The listing builds one solid part. Answer for the finished solid, in the listing's coordinates (mm). Face numbers are marked on the shaded views. A direction names the side the tool comes from. Give positions to 0.01 mm unless a question says otherwise; leave off trailing zeros. Loops run counter-clockwise (first coordinate to the right, second up) from the corner with the lowest first, then second, coordinate; pieces in that order, holes last. Notation, with made-up numbers: (42.25, -18) - (73.25, -18) arc R15 cw to (73.25, 11) - close; hole circle Ø8 at (85, 51). An arc over 180 degrees is marked (long way). Answer in a Markdown table with one row per item. Add a question column.
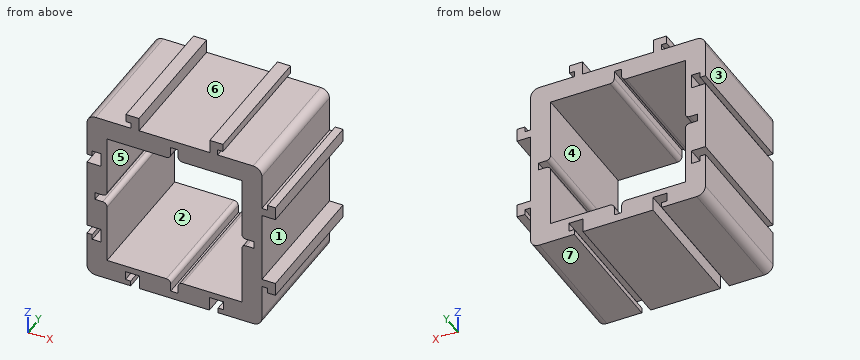
```python
from build123d import *

# Parameters (mm, degrees)
SKETCH1_W           = 50.8
SKETCH1_H           = 50.8
BOSS_EXTRUDE1_DEPTH = 38.1
FILLET1_R           = 2.54
FILLET2_R           = 1.27
SKETCH3_W           = 1.524
SKETCH3_H           = 2.54
SKETCH3_W_2         = 2.54
SKETCH3_H_2         = 1.524
CUT_EXTRUDE1_DEPTH  = 53.363441445
SKETCH5_W           = 2.286
SKETCH5_H           = 2.286
SKETCH5_H_2         = 1.651
SKETCH5_W_2         = 1.524
SKETCH5_H_3         = 1.524
SKETCH5_W_3         = 1.651
BOSS_EXTRUDE2_DEPTH = 38.1


with BuildPart() as part:
    # Sketch1 → Boss-Extrude1 (new body)
    with BuildSketch(Plane(origin=(0, 0, 0), x_dir=(1, 0, 0), z_dir=(0, 1, 0))):
        Rectangle(SKETCH1_W, SKETCH1_H)
        Polygon((-1.0795, -19.558), (-1.0795, -23.114), (1.0795, -23.114), (1.0795, -19.558), (19.558, -19.558), (19.558, -1.0795), (23.114, -1.0795), (23.114, 1.0795), (19.558, 1.0795), (19.558, 19.558), (1.0795, 19.558), (1.0795, 23.114), (-1.0795, 23.114), (-1.0795, 19.558), (-19.558, 19.558), (-19.558, 1.0795), (-23.114, 1.0795), (-23.114, -1.0795), (-19.558, -1.0795), (-19.558, -19.558), align=None, mode=Mode.SUBTRACT)
    extrude(amount=BOSS_EXTRUDE1_DEPTH)

    # Fillet1
    fillet1_edges = [part.edges().sort_by_distance(p)[0] for p in [
        (-25.4, 19.05, -25.4),
        (25.4, 19.05, -25.4),
        (25.4, 19.05, 25.4),
        (-25.4, 19.05, 25.4),
    ]]
    fillet(fillet1_edges, radius=FILLET1_R)

    # Fillet2
    fillet2_edges = [part.edges().sort_by_distance(p)[0] for p in [
        (1.0795, 19.05, 19.558),
        (19.558, 19.05, 1.0795),
        (19.558, 19.05, -1.0795),
        (1.0795, 19.05, -19.558),
        (-1.0795, 19.05, -19.558),
        (-19.558, 19.05, -1.0795),
        (-19.558, 19.05, 1.0795),
        (-1.0795, 19.05, 19.558),
    ]]
    fillet(fillet2_edges, radius=FILLET2_R)

    # Sketch3 → Cut-Extrude1 (cut, through all)
    with BuildSketch(Plane(origin=(0, 38.1, 0), x_dir=(1, 0, 0), z_dir=(0, 1, 0))):
        with Locations((-24.638, 11.43)):
            Rectangle(SKETCH3_W, SKETCH3_H)
        with Locations((-22.606, 11.43)):
            Rectangle(SKETCH3_W_2, SKETCH3_H)
        with Locations((-22.606, 13.462)):
            Rectangle(SKETCH3_W_2, SKETCH3_H_2)
        with Locations((-24.638, -11.43)):
            Rectangle(SKETCH3_W, SKETCH3_H)
        with Locations((-22.606, -11.43)):
            Rectangle(SKETCH3_W_2, SKETCH3_H)
        with Locations((-22.606, -13.462)):
            Rectangle(SKETCH3_W_2, SKETCH3_H_2)
        with Locations((-11.43, 24.638)):
            Rectangle(SKETCH3_W_2, SKETCH3_H_2)
        with Locations((-11.43, 22.606)):
            Rectangle(SKETCH3_W_2, SKETCH3_H)
        with Locations((-13.462, 22.606)):
            Rectangle(SKETCH3_W, SKETCH3_H)
        with Locations((11.43, 24.638)):
            Rectangle(SKETCH3_W_2, SKETCH3_H_2)
        with Locations((11.43, 22.606)):
            Rectangle(SKETCH3_W_2, SKETCH3_H)
        with Locations((13.462, 22.606)):
            Rectangle(SKETCH3_W, SKETCH3_H)
    extrude(amount=-CUT_EXTRUDE1_DEPTH, mode=Mode.SUBTRACT)

    # Sketch5 → Boss-Extrude2 (add)
    with BuildSketch(Plane(origin=(0, 38.1, 0), x_dir=(1, 0, 0), z_dir=(0, 1, 0))):
        with Locations((-11.43, -28.194)):
            Rectangle(SKETCH5_W, SKETCH5_H)
        with Locations((-11.43, -26.2255)):
            Rectangle(SKETCH5_W, SKETCH5_H_2)
        with Locations((-13.335, -28.194)):
            Rectangle(SKETCH5_W_2, SKETCH5_H)
        with Locations((11.43, -28.194)):
            Rectangle(SKETCH5_W, SKETCH5_H)
        with Locations((13.335, -28.194)):
            Rectangle(SKETCH5_W_2, SKETCH5_H)
        with Locations((11.43, -26.2255)):
            Rectangle(SKETCH5_W, SKETCH5_H_2)
        with Locations((28.194, -11.43)):
            Rectangle(SKETCH5_W, SKETCH5_H)
        with Locations((28.194, -13.335)):
            Rectangle(SKETCH5_W, SKETCH5_H_3)
        with Locations((26.2255, -11.43)):
            Rectangle(SKETCH5_W_3, SKETCH5_H)
        with Locations((28.194, 13.335)):
            Rectangle(SKETCH5_W, SKETCH5_H_3)
        with Locations((28.194, 11.43)):
            Rectangle(SKETCH5_W, SKETCH5_H)
        with Locations((26.2255, 11.43)):
            Rectangle(SKETCH5_W_3, SKETCH5_H)
    extrude(amount=-BOSS_EXTRUDE2_DEPTH)


solid = part.part
```
(1) A tool of negligible diameter and unlimited length cuts with its end or side. For the marked faces 1, 2 and 3, from which of +Z, -Z, +X, -X, +Y, -Y can it reach the whole face along a straight path? Write none if from no direction.
(2) A cutting plane is placed at B-B on z = 11. Determine the outline of the cut face in (x, y), plus the area to 3 significant figures.
(3) Given pin 1 Ø0.7 at (y, z) = (10, -22.5) entering from +X; pin 2 Ø8 at (x, z) = (9, 15.5) entering from -Y; pin 3 Ø1.2 at (x, y) = (-25, 26.5) entering from -Z; pin 4 Ø4.5 at (x, y) = (-23.5, 27.5) entering from +Z, each flat-ended and moving along its own axis, determine where each tip first touches the part or whether it passes through.
(4) The mould has two halves that part along Z. Classify the marked faces 4, 5, 6 and 7: pulls with the +Z half, pulls with the -Z half, needs draft (parallel to the pull), parting line crosses it, or undercut.
(5) A cutting plane is placed at A-A on x = -15. Determine the outline of the cut face in (y, z), plus the area to 3 significant figures.
(6) Find the intervals of material crossed by line 1 along Z through (x, y) = (18, 10); line 2 along X through (y, z) = (7, 14), in increasing order. Write a range as [from, to].
Evaluation:
| question | item | result |
|---|---|---|
| 1 | face 1 | +X, +Y, -Y |
| 1 | face 2 | +Y, -Y |
| 1 | face 3 | +Z, -Z, -X, +Y, -Y |
| 2 | outline | (-21.34, 0) - (-19.56, 0) - (-19.56, 38.1) - (-21.34, 38.1) - close; (19.56, 0) - (29.34, 0) - (29.34, 38.1) - (19.56, 38.1) - close |
| 2 | area | 440 mm² |
| 3 | pin 1 | stops at x = 25.4 |
| 3 | pin 2 | passes through |
| 3 | pin 3 | stops at z = -24.88 |
| 3 | pin 4 | stops at z = 25.4 |
| 4 | face 4 | undercut |
| 4 | face 5 | undercut |
| 4 | face 6 | pulls with the +Z half |
| 4 | face 7 | pulls with the -Z half |
| 5 | outline | (0, -25.4) - (38.1, -25.4) - (38.1, -19.56) - (0, -19.56) - close; (0, 19.56) - (38.1, 19.56) - (38.1, 25.4) - (0, 25.4) - close |
| 5 | area | 445 mm² |
| 6 | line 1 | z = [-25.4, -19.56], [19.56, 25.4] |
| 6 | line 2 | x = [-25.4, -23.88], [-21.34, -19.56], [19.56, 25.4], [27.05, 29.34] |
